Part model, mm, in its own coordinate system. A direction names the side the tool comes from. Coordinates: 2 decimals unless noted, no trailing zeros. Loops run counter-clockwise (first coordinate to the right, second up) from the corner with the lowest first, then second, coordinate; pieces in that order, holes last. Notation, with made-up numbers: (89.5, 39) -> (111.5, 39) arc R20 ccw to (111.5, 53) -> close; hole circle Ø4 at (12, -39). An arc over 180 degrees is marked (long way). Use one line per item in the form item = value. Start each with the question number.
(1) Drill centre lines: L1, parallel to Y at x = -3.75, z = 15; L2, parallel to Y at x = 5.5, z = 10.25; L3, parallel to Z at x = 8, y = -3.75. Where is each one in solid material? Low to high. Write a range as [from, to].
(2) Band-saw the part on A-A on y = 0. Give the cut face in (x, z), then the cut area to 3 significant figures.
(3) Band-saw the part on D-D on y = -6. Give the cut face in (x, z), then the cut area to 3 significant figures.
(4) 3-axis set-ups, long thin cutter, end or side, ignore diameter. For faces 1 (the flat face through (13, 0, -5.303)), 2 (the flat face through (2, 3, 2)), 3 (the flat face through (-5.303, 0, 13)): which of +Z, -Z, +X, -X, +Y, -Y reach the whole face in a straight line?
(5) Mould opens along Z. For faces 4 (the flat face through (9, 5, 13)), 5 (the cylindrical face through (16.5, 0.07, -3.82)), 6 (the cylindrical face through (-0.92, 0.04, 1.03)) say: +Z half, -Z half, draft (parallel to the pull), parting line (faces both ways), or undercut.
(6) Band-saw the part on C-C on x = 0.5. Count the separate pieces of the cut face and the enclosed holes in it, then the cut area to 3 significant figures.
(7) Pin check, flat tips, straight feed: P1, Ø1.8, axis at x = 15, y = 0, coming from the +Z side; P2, Ø1.5, axis at x = 14.5, y = 0, coming from the -Z side; P3, Ø1.8, axis at x = 16.5, y = 1.5, coming from the -Z side. Stop position of each tip, or through.
(8) Band-saw the part on B-B on x = 17.5. Give the cut face in (y, z), then the cut area to 3 significant figures.
```python
from build123d import *

# Parameters (mm, degrees)
BOSS_EXTRUDE1_DEPTH = 3
SKETCH2_R           = 7.5
SKETCH2_R_2         = 5.075
BOSS_EXTRUDE2_DEPTH = 12.02
SKETCH3_R           = 5.075
CUT_EXTRUDE1_DEPTH  = 12.02
SKETCH4_R           = 1.5
CUT_EXTRUDE2_DEPTH  = 6
SKETCH5_R           = 1.5
CUT_EXTRUDE3_DEPTH  = 3
SKETCH6_R           = 1.5
CUT_EXTRUDE4_DEPTH  = 3


with BuildPart() as part:
    # Sketch1 → Boss-Extrude1 (new, symmetric)
    with BuildSketch(Plane(origin=(0, 0, 0), x_dir=(1, 0, 0), z_dir=(0, 1, 0))):
        with BuildLine():
            Line((20.5, -1.5), (20.5, 0))
            Line((20.5, 0), (20.5, 2.035533906))
            Line((20.5, 2.035533906), (20.5, 3.535533906))
            Line((20.5, 3.535533906), (20.5, 5.303300859))
            Line((20.5, 5.303300859), (5.303300859, 5.303300859))
            ThreePointArc((5.303300859, 5.303300859), (-2.828427125, 2.828427125), (-5.303300859, -5.303300859))
            Line((-5.303300859, -5.303300859), (-5.303300859, -20.5))
            Line((-5.303300859, -20.5), (-3.535533906, -20.5))
            Line((-3.535533906, -20.5), (-2.035533906, -20.5))
            Line((-2.035533906, -20.5), (0, -20.5))
            Line((0, -20.5), (1.5, -20.5))
            Line((1.5, -20.5), (20.5, -1.5))
        make_face()
    extrude(amount=BOSS_EXTRUDE1_DEPTH, both=True)

    # Sketch2 → Boss-Extrude2 (add)
    with BuildSketch(Plane(origin=(11, 0, 11), x_dir=(0.7071067811865475, 0, -0.7071067811865477), z_dir=(0.7071067811865477, 0, 0.7071067811865475))):
        Circle(SKETCH2_R)
        Circle(SKETCH2_R_2, mode=Mode.SUBTRACT)
    extrude(amount=-BOSS_EXTRUDE2_DEPTH)

    # Sketch3 → Cut-Extrude1 (cut)
    with BuildSketch(Plane(origin=(11, 0, 11), x_dir=(0.7071067811865475, 0, -0.7071067811865477), z_dir=(0.7071067811865477, 0, 0.7071067811865475))):
        Circle(SKETCH3_R)
    extrude(amount=-CUT_EXTRUDE1_DEPTH, mode=Mode.SUBTRACT)

    # Sketch4 → Cut-Extrude2 (cut)
    with BuildSketch(Plane(origin=(0, 3, 0), x_dir=(1, 0, 0), z_dir=(0, 1, 0))):
        with Locations(Location((-0.349848925, 0.357263409, 0), (0, 0, 270))):
            Circle(SKETCH4_R)
    extrude(amount=-CUT_EXTRUDE2_DEPTH, mode=Mode.SUBTRACT)

    # Sketch5 → Cut-Extrude3 (cut)
    with BuildSketch(Plane.ZY.offset(5.303300859)):
        with Locations((15, 0)):
            Circle(SKETCH5_R)
    extrude(amount=-CUT_EXTRUDE3_DEPTH, mode=Mode.SUBTRACT)

    # Sketch6 → Cut-Extrude4 (cut)
    with BuildSketch(Plane(origin=(0, 0, -5.303300859), x_dir=(-1, 0, 0), z_dir=(0, 0, -1))):
        with Locations((-15, 0)):
            Circle(SKETCH6_R)
    extrude(amount=-CUT_EXTRUDE4_DEPTH, mode=Mode.SUBTRACT)


solid = part.part
```
A:
q1.L1 = [-3, -1.5], [1.5, 3]
q1.L2 = [-6.71, -3.8], [3.8, 6.71]
q1.L3 = [-1.19, 3.16], [12.84, 14]
q2.outline = (-5.3, 5.3) arc R9.03 ccw to (5.3, -5.3) -> (13.5, -5.3) -> (13.5, -2.3) -> (16.5, -2.3) -> (16.5, -5.3) -> (20.5, -5.3) -> (20.5, 1.5) -> (14.59, 7.41) -> (6.09, -1.09) -> (-1.09, 6.09) -> (7.41, 14.59) -> (1.5, 20.5) -> (-5.3, 20.5) -> (-5.3, 16.5) -> (-2.3, 16.5) -> (-2.3, 13.5) -> (-5.3, 13.5) -> close; hole circle Ø3 at (-0.35, -0.36)
q2.area = 324 mm²
q3.outline = (-0.68, 5.68) -> (5.68, -0.68) -> (14.18, 7.82) -> (7.82, 14.18) -> close
q3.area = 108 mm²
q4.face_1 = -Z, +X, +Y, -Y
q4.face_2 = +Y
q4.face_3 = +Z, -X, +Y, -Y
q5.face_4 = +Z half
q5.face_5 = draft
q5.face_6 = undercut
q6.separate_pieces = 3
q6.enclosed_holes = 0
q6.area = 147 mm²
q7.P1 = 7.45
q7.P2 = -2.3
q7.P3 = -5.3
q8.outline = (-3, -5.3) -> (3, -5.3) -> (3, 4.5) -> (-3, 4.5) -> close
q8.area = 58.8 mm²
